Could you check a few things on this drawing? It's one solid part, dimensions in mm from its lowest x, y, z. A direction names the side the tool comes from. Round coordinates to 2 decimals unless told otherwise and drop trailing zeros. Write each loop counter-clockwise with the first axis right and the second up, starting at its lowest first coordinate (ties: lowest second). Pieces come first, ordered by that corner, then holes. Notation, with made-up numbers: (70.5, 62) - (78.5, 62) arc R33 cw to (78.5, 90) - close; hole circle Ø9 at (-32, 52). An arc over 180 degrees is marked (long way). Write item = value, one per line. Start each with the question number.
Item 1: Thinking about a two-plate mould opening in X: for the marked faces 3, 4 and 5, which applies, pulls with the +X half, pulls with the -X half, needs draft (parallel to the pull), parting line crosses it, or undercut?
Item 2: Which directions (+Z, -Z, +X, -X, +Y, -Y) give clear straight access to the entire face, cutting with the end or side of a thin tool? Please do the marked faces 1 and 2.
Item 3: If we section it at D-D (y = 18): Please give me the cut outline in (x, z), and give its area (3 significant figures).
Item 4: For P1, Ø2, axis at x = 21, z = 11.5, coming from the +Y side, with a flat end and sliding along its axis, tell me the tip position at first contact or that it passes through.
Item 5: If we section it at A-A (y = 8.75): Please give me the cut outline in (x, z).
Item 6: If we section it at C-C (z = 11.5): Please give me the cut outline in (x, y).
Item 7: If we section it at B-B (x = 2.85): Please give me the cut outline in (y, z).
Item 8: If I drill on line 1 along X through (y, z) = (12.75, 1); line 2 along Y through (x, z) = (8.5, 11.5); line 3 along Z through (x, y) = (32.35, 1), over which ranges is the centre line in solid material (lowest first)? Write a range as [from, to].
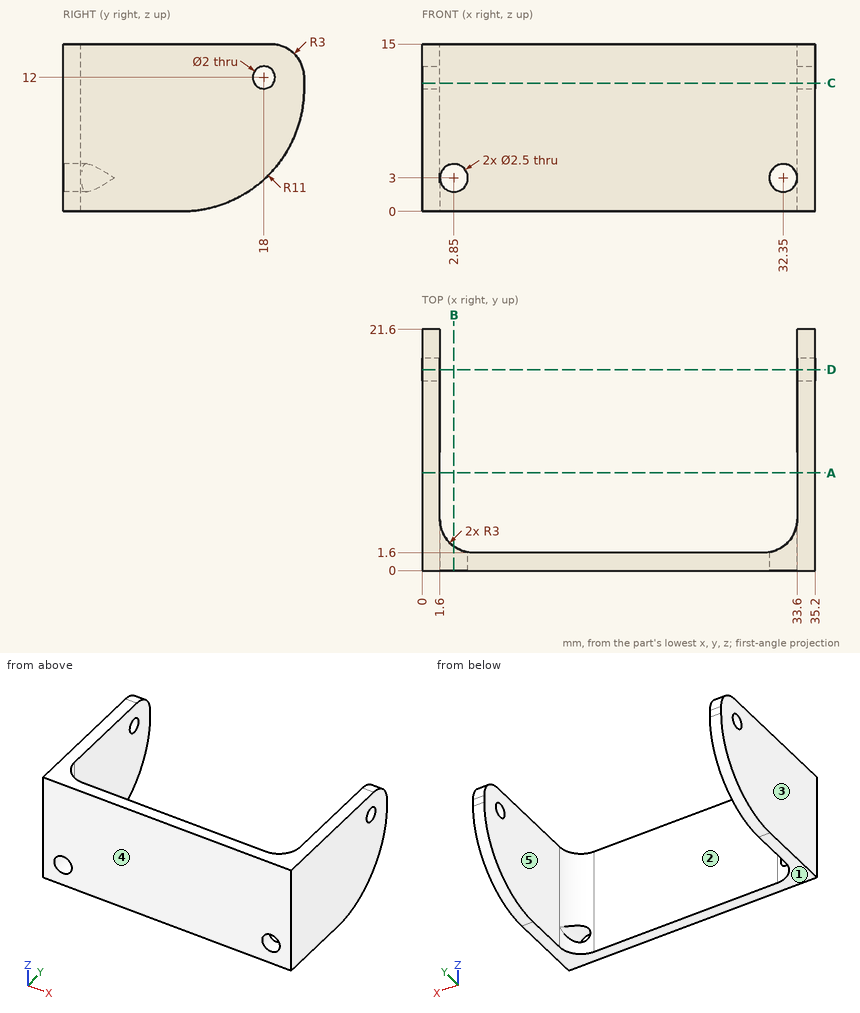
Reply:
q1.face_3 = pulls with the -X half
q1.face_4 = needs draft
q1.face_5 = undercut
q2.face_1 = -Z, +X, -X, +Y, -Y
q2.face_2 = +Z, -Z, +Y
q3.outline = (0, 2.86) - (1.6, 2.86) - (1.6, 11) - (0, 11) - close; (0, 13) - (1.6, 13) - (1.6, 15) - (0, 15) - close; (33.6, 2.86) - (35.2, 2.86) - (35.2, 11) - (33.6, 11) - close; (33.6, 13) - (35.2, 13) - (35.2, 15) - (33.6, 15) - close
q3.area = 32.4 mm2
q4.P1 = 1.6
q5.outline = (0, 0) - (1.6, 0) - (1.6, 15) - (0, 15) - close; (33.6, 0) - (35.2, 0) - (35.2, 15) - (33.6, 15) - close
q6.outline = (0, 0) - (35.2, 0) - (35.2, 17.13) - (33.6, 17.13) - (33.6, 4.6) arc R3 cw to (30.6, 1.6) - (4.6, 1.6) arc R3 cw to (1.6, 4.6) - (1.6, 17.13) - (0, 17.13) - close; (0, 18.87) - (1.6, 18.87) - (1.6, 21.6) - (0, 21.6) - close; (33.6, 18.87) - (35.2, 18.87) - (35.2, 21.6) - (33.6, 21.6) - close
q7.outline = (0, 0) - (2.16, 0) - (2.16, 1.75) - (0, 1.75) - close; (0, 4.25) - (2.16, 4.25) - (2.16, 15) - (0, 15) - close
q8.line_1 = [0, 1.6], [33.6, 35.2]
q8.line_2 = [0, 1.6]
q8.line_3 = [0, 1.75], [4.25, 15]
